from build123d import *

# Parameters (mm, degrees)
F0_W     = 901.7
F0_H     = 584.2
F1_DEPTH = 88.9
F2_R     = 76.2
F3_W     = 825.5
F3_H     = 508
F4_DEPTH = 3.175
F6_DEPTH = 1.27


with BuildPart() as f1:
    # F0 (on Front) → F1 (new body)
    with BuildSketch(Plane.XZ):
        Rectangle(F0_W, F0_H)
    extrude(amount=-F1_DEPTH)

    # F2
    f2_edges = [f1.edges().sort_by_distance(p)[0] for p in [
        (0, 88.9, 292.1),
        (-450.85, 88.9, 0),
        (0, 88.9, -292.1),
        (450.85, 88.9, 0),
    ]]
    fillet(f2_edges, radius=F2_R)

    # F3 (on face) → F4 (cut)
    with BuildSketch(Plane.XZ):
        Rectangle(F3_W, F3_H)
    extrude(amount=-F4_DEPTH, mode=Mode.SUBTRACT)

    # F5 (on Right) → F6 (join, symmetric)
    with BuildSketch(Plane.YZ):
        Polygon((88.9, -307.528856), (187.325, 259.589197), (88.9, 276.671144), align=None)
    extrude(amount=F6_DEPTH, both=True)


solid = f1.part
Could you check a few things on this model? Use its own coordinates, in mm. A direction names the side the tool comes from. Coordinates: 2 decimals unless noted, no trailing zeros. Write each loop counter-clockwise with the first axis right and the second up, starting at its lowest first coordinate (ties: lowest second). Pieces come first, ordered by that corner, then holes. Notation, with made-up numbers: M 14,58 L 21,58 A23 ccw 21,88 Z; hole C -14,13.25 d2. An arc over 180 degrees is marked long. One line per question, with ' | ' between items.
1) Imagine slicing it at D-D, the plane z = -135. Write out the boundary of the cut face in (x, y) (3 decimals).
Checks:
outline: M -450.85,0 L -412.75,0 L -412.75,3.175 L 412.75,3.175 L 412.75,0 L 450.85,0 L 450.85,12.7 A76.2 ccw 374.65,88.9 L 1.27,88.9 L 1.27,118.843 L -1.27,118.843 L -1.27,88.9 L -374.65,88.9 A76.2 ccw -450.85,12.7 Z
2) If we mould it in two halves opening along X, with no side actions, what happens to faces 1 (the face through (6.312, 65.986, 270.371)), 2 (the face through (-429.121, 65.986, 4.089)), 3 (the face through (-6, 3.175, 4)), 4 (the face through (429.121, 65.986, 4.089))? For each: released by +X, released by -X, zero draft, split by the parting line, or undercut.
Checks:
face 1: zero draft | face 2: released by -X | face 3: undercut | face 4: released by +X
3) Imagine slicing it at A-A, the plane x = -18.5. Write out the boundary of the cut face in (y, z) (3 decimals).
Checks:
outline: M 0,-292.1 L 12.7,-292.1 A76.2 ccw 88.9,-215.9 L 88.9,215.9 A76.2 ccw 12.7,292.1 L 0,292.1 L 0,254 L 3.175,254 L 3.175,-254 L 0,-254 Z
4) For pin 1 Ø2 at (y, z) = (106.5, -195.5) entering from -X; pin 2 Ø12 at (y, z) = (49, 4.5) entering from -X; pin 3 Ø6.5 at (x, y) = (9.5, 4) entering from -Z, each with a flat end and sliding along its axis, tell me the tip position at first contact or that it passes through.
Checks:
pin 1: x = -1.27 | pin 2: x = -444.57 | pin 3: z = -292.1
5) I need wall thicknesses on probe 1 along Y at (x, z) = (-342, 40.5) (3 decimals); probe 2 along Z at (x, y) = (132, 11); probe 3 along Y at (x, z) = (-378.5, 30) (3 decimals). Which ranges of each line are inside material? Lowest first, please. Write a range as [from, to].
Checks:
probe 1: [3.175, 88.9] | probe 2: [-292.1, 292.1] | probe 3: [3.175, 88.803]
6) For faces 5 (the face through (0.018, 137.424, -27.94)), 6 (the face through (-1.27, 126, 54)), 7 (the face through (185, 88.9, 3)), which set-ups out of +Z, -Z, +X, -X, +Y, -Y let a thin tool reach every point of the face, with its end or its side?
Checks:
face 5: -Z, +X, -X, +Y | face 6: +Z, -Z, -X, +Y | face 7: +Z, -Z, +X, +Y
7) Imagine slicing it at C-C, the plane y = 157. Write out the boundary of the cut face in (x, z).
Checks:
outline: M -1.27,84.86 L 1.27,84.86 L 1.27,264.85 L -1.27,264.85 Z
8) Imagine slicing it at B-B, the plane z = 77.5. Write out the boundary of the cut face in (x, y) (3 decimals), and give its area (3 significant figures).
Checks:
outline: M -450.85,0 L -412.75,0 L -412.75,3.175 L 412.75,3.175 L 412.75,0 L 450.85,0 L 450.85,12.7 A76.2 ccw 374.65,88.9 L 1.27,88.9 L 1.27,155.723 L -1.27,155.723 L -1.27,88.9 L -374.65,88.9 A76.2 ccw -450.85,12.7 Z | area: 75,200 mm²
